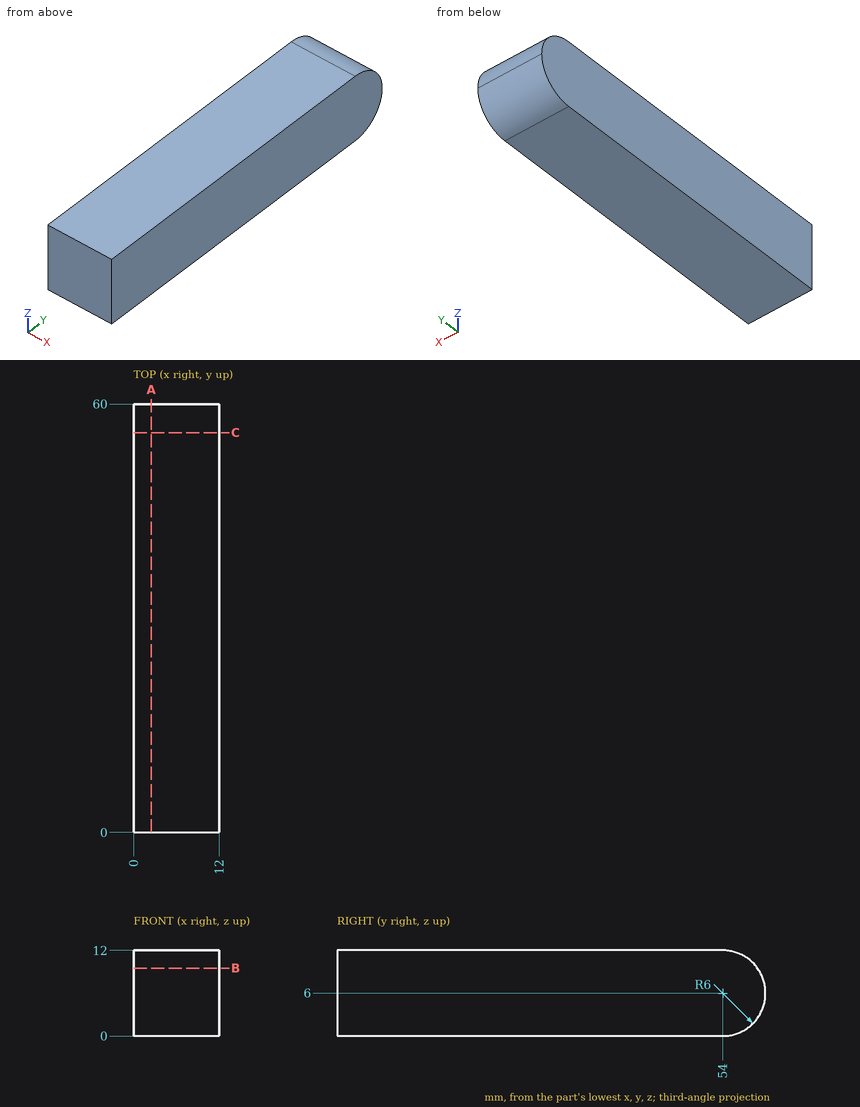
Could you check a few things on this drawing? It's one solid part, dimensions in mm from its lowest x, y, z. Round coordinates to 2 decimals unless told otherwise and drop trailing zeros. Loops run counter-clockwise (first coordinate to the right, second up) from the corner with the lowest first, then second, coordinate; pieces in that order, holes last. Notation, with made-up numbers: (-31.5, 53) -> (-6.5, 53) arc R20 ccw to (-6.5, 68) -> close; hole circle Ø4 at (37, -23). An arc over 180 degrees is marked (long way). One line per item, written item: value. Start each with the question number.
1. If we section it at B-B, the plane z = 9.5: Write out the boundary of the cut face in (x, y).
2. For pin 1 (4 mm diameter, centred on y = 50, z = 3, fed in from -X), with a flat end and sliding along its axis, tell me the tip position at first contact or that it passes through.
3. If we section it at C-C, the plane y = 56: Write out the boundary of the cut face in (x, z), then the cut area to 3 significant figures.
4. If we section it at A-A, the plane x = 2.5: Write out the boundary of the cut face in (y, z).
5. If I drill on probe 1 along Y at (x, z) = (10.75, 6.5); probe 2 along Y at (x, z) = (4.5, 10); probe 3 along Z at (x, y) = (9.75, 57.5), over which ranges is the centre line in solid material (lowest first)?
Calculated:
1. outline: (0, 0) -> (12, 0) -> (12, 58.87) -> (0, 58.87) -> close
2. pin 1: stops at x = 0
3. outline: (0, 0.34) -> (12, 0.34) -> (12, 11.66) -> (0, 11.66) -> close
3. area: 136 mm²
4. outline: (0, 0) -> (54, 0) arc R6 ccw to (60, 6) arc R6 ccw to (54, 12) -> (0, 12) -> close
5. probe 1: y = 0 to 59.98
5. probe 2: y = 0 to 58.47
5. probe 3: z = 1.13 to 10.87
